Input: part model. Units: mm. Frame: model coordinates. A direction names the side the tool comes from. Coordinates: 2 decimals unless noted, no trailing zeros. Write each loop counter-clockwise with the first axis right and the second up, starting at its lowest first coordinate (ties: lowest second). Pieces come first, ordered by that corner, then holes.
1) Set-up query: faces 5 (the flat face through (-11, 22.585, 21)), 6 (the flat face through (12.7, -57, 2)), 7 (the flat face through (43, -6.35, 21)). Return all of +Z, -Z, +X, -X, +Y, -Y with unobstructed straight access to the full face (end or side cutting, diameter ignored); none if empty.
2) Section query C-C (y = -21.5). Output: boundary loops of the cut face in (x, z), then the cut area to 3 significant figures.
3) Section query D-D (x = -3.5). Output: boundary loops of the cut face in (y, z), then the cut area to 3 significant figures.
4) Draft query along X for faces 1 (the flat face through (-12.7, -57, 2)), 2 (the flat face through (-13, 20.045, 21)), 3 (the flat face through (40.333, 6.631, 18.157)), 4 (the flat face through (-31, -25.4, 2)). Return one class per face: pulls with the +X half, pulls with the -X half, needs draft (parallel to the pull), parting line crosses it, or undercut.
5) Section query A-A (z = 35). State how many separate pieces and enclosed holes the cut face has, then the cut area to 3 significant figures.
6) Pin query (flat end, axial travel): pin 1 Ø4 at (y, z) = (-52.5, 2.5) entering from +X; pin 2 Ø8 at (x, z) = (42.5, 19.5) entering from -Y; pin 3 Ø8 at (x, z) = (-26, 11) entering from +Y; pin 4 Ø2 at (y, z) = (-65.5, 6.5) entering from -X. Return the tip coordinate at first contact, or that it passes through.
7) Section query B-B (x = 36). Output: boundary loops of the cut face in (y, z).
8) Line query: L1, parallel to Y at x = 8, z = 17; L2, parallel to Z at x = -8.5, y = -48.5; L3, parallel to Y at x = -6.5, z = 7.5. Output: solid intervals per line, ascending.
from build123d import *

# Parameters (mm, degrees)
F1_DEPTH  = 36.83
F3_DEPTH  = 33.02
F5_DEPTH  = 33.02
F6_R      = 0.635
F7_DEPTH  = 6.35
F9_R      = 0.635
F10_DEPTH = 6.35
F8_R      = 0.635
F11_DEPTH = 6.35
F12_W     = 25.4
F12_H     = 63.5
F13_DEPTH = 3.81


with BuildPart() as f1:
    # F0 (on Top) → F1 (new body)
    with BuildSketch(Plane.XY):
        Polygon((-19.05, 24.4902079291), (-48.2362932828, 0), (-48.2362932828, -25.4), (48.2362932828, -25.4), (48.2362932828, 0), (19.05, 24.4902079291), align=None)
    extrude(amount=F1_DEPTH)

    # F2 (on face) → F3 (cut)
    with BuildSketch(Plane.XY.offset(36.83)):
        Polygon((-16.7387890124, 18.1402079291), (-38.3574469823, 0), (-38.3574469823, -6.35), (-48.2362932828, -6.35), (-48.2362932828, -25.4), (-38.3574469823, -25.4), (38.3574469823, -25.4), (48.2362932828, -25.4), (48.2362932828, -6.35), (38.3574469823, -6.35), (38.3574469823, 0), (16.7387890124, 18.1402079291), align=None)
    extrude(amount=-F3_DEPTH, mode=Mode.SUBTRACT)

    # F4 (on face) → F5 (cut)
    with BuildSketch(Plane.XY.offset(36.83)):
        Polygon((15.875, 22.5852079291), (6.35, 22.5852079291), (6.35, 24.4902079291), (-6.35, 24.4902079291), (-6.35, 22.5852079291), (-15.875, 22.5852079291), (-15.875, 20.0452079291), (-9.525, 20.0452079291), (-9.525, 18.1402079291), (3.175, 18.1402079291), (3.175, 20.0452079291), (15.875, 20.0452079291), align=None)
        Polygon((22.2648719992, 13.503273733), (31.9936364268, 5.33987109), (33.2181468233, 6.7991857541), (42.9469112509, -1.3642168889), (44.5795917795, 0.5815359966), (37.2830184588, 6.7040879789), (38.5075288552, 8.163402643), (28.7787644276, 16.326805286), (27.5542540312, 14.8674906219), (20.2576807104, 20.9900426042), (18.6250001818, 19.0442897186), (23.4893823957, 14.9625883971), align=None)
        Polygon((-42.9469112509, -1.3642168889), (-38.0825290371, 2.7174844326), (-36.8580186406, 1.2581697685), (-27.129254213, 9.4215724115), (-28.3537646095, 10.8808870756), (-18.6250001818, 19.0442897186), (-20.2576807104, 20.9900426042), (-27.5542540312, 14.8674906219), (-28.7787644276, 16.326805286), (-38.5075288552, 8.163402643), (-37.2830184588, 6.7040879789), (-44.5795917795, 0.5815359966), align=None)
    extrude(amount=-F5_DEPTH, mode=Mode.SUBTRACT)

    # F6 (on face) → F7 (cut, through all)
    with BuildSketch(Plane(origin=(-19.9300744284, 23.7517378008, 0), x_dir=(-0.7660444431, -0.6427876097, 0), z_dir=(-0.6427876097, 0.7660444431, 0))):
        with Locations((6.788644426, 19.685)):
            Circle(F6_R)
        with Locations((29.013644426, 19.685)):
            Circle(F6_R)
    extrude(amount=-F7_DEPTH, mode=Mode.SUBTRACT)

    # F9 (on face) → F10 (cut, through all)
    with BuildSketch(Plane(origin=(19.9300744284, 23.7517378008, 0), x_dir=(-0.7660444431, 0.6427876097, 0), z_dir=(0.6427876097, 0.7660444431, 0))):
        with Locations((-29.013644426, 19.685)):
            Circle(F9_R)
        with Locations((-6.788644426, 19.685)):
            Circle(F9_R)
    extrude(amount=-F10_DEPTH, mode=Mode.SUBTRACT)

    # F8 (on face) → F11 (cut, through all)
    with BuildSketch(Plane(origin=(0, 24.4902079291, 0), x_dir=(-1, 0, 0), z_dir=(0, 1, 0))):
        with Locations((-11.1125, 19.685)):
            Circle(F8_R)
        with Locations((11.1125, 19.685)):
            Circle(F8_R)
    extrude(amount=-F11_DEPTH, mode=Mode.SUBTRACT)

    # F12 (on face) → F13 (join, through all)
    with BuildSketch(Plane(origin=(0, 0, 0), x_dir=(1, 0, 0), z_dir=(0, 0, -1))):
        with Locations((0, 57.15)):
            Rectangle(F12_W, F12_H)
    extrude(amount=-F13_DEPTH)


solid = f1.part
Answer:
1. face 5: +Z
1. face 6: +Z, -Z, +X, -Y
1. face 7: +Z, +X, -X, -Y
2. outline: (-48.24, 0) - (48.24, 0) - (48.24, 3.81) - (-48.24, 3.81) - close
2. area: 368 mm2
3. outline: (-88.9, 0) - (24.49, 0) - (24.49, 3.81) - (-88.9, 3.81) - close
3. area: 432 mm2
4. face 1: pulls with the -X half
4. face 2: undercut
4. face 3: pulls with the +X half
4. face 4: needs draft
5. separate pieces: 4
5. enclosed holes: 0
5. area: 387 mm2
6. pin 1: stops at x = 12.7
6. pin 2: stops at y = -6.35
6. pin 3: stops at y = 22.01
6. pin 4: passes through
7. outline: (-25.4, 0) - (10.27, 0) - (10.27, 3.81) - (4.46, 3.81) - (4.46, 36.83) - (1.98, 36.83) - (1.98, 3.81) - (-25.4, 3.81) - close
8. L1: y = 18.14 to 20.05, 22.59 to 24.49
8. L2: z = 0 to 3.81
8. L3: y = 22.59 to 24.49
